```python
from build123d import *

# Parameters (mm, degrees)
F1_DEPTH  = 76.2
F2_R      = 26.962809
F3_DEPTH  = 63.798865
F5_DEPTH  = 127
F7_DEPTH  = 127
F8_R      = 8.119413
F9_DEPTH  = 48.922082
F10_R     = 9.932107
F11_DEPTH = 52.600686


with BuildPart() as f1:
    # F0 (on Front) → F1 (new body)
    with BuildSketch(Plane.XZ):
        Polygon((-32.091218, -26.459824), (-32.091218, -51.57762), (56.808782, -51.57762), (56.808782, -26.17762), (31.408782, -26.17762), (31.408782, 37.32238), (56.808782, 37.32238), (56.808782, 62.72238), (-32.389083, 62.72238), (-32.091218, 35.914471), (-7.385746, 36.188975), (-6.692785, -26.17762), align=None)
    extrude(amount=F1_DEPTH)

    # F2 (on face) → F3 (cut, through all)
    with BuildSketch(Plane.YZ.offset(31.408782)):
        with Locations((-38.1, 5.57238)):
            Circle(F2_R)
    extrude(amount=-F3_DEPTH, mode=Mode.SUBTRACT)

    # F4 (on face) → F5 (join)
    with BuildSketch(Plane.XY.offset(62.72238)):
        Polygon((5.720465, -23.600314), (7.3049, -48.921082), (38.345255, -48.921082), (38.345255, -23.600314), align=None)
    extrude(amount=F5_DEPTH)

    # F6 (on face) → F7 (join)
    with BuildSketch(Plane.XY.offset(62.72238)):
        Polygon((-2.503503, -46.93903), (-10.301619, -21.702323), (-23.880914, -20.912418), (-23.880914, -46.93903), align=None)
    extrude(amount=F7_DEPTH)

    # F8 (on face) → F9 (cut, through all)
    with BuildSketch(Plane.XZ.offset(48.921082)):
        with Locations((21.437701, 170.965254)):
            Circle(F8_R)
    extrude(amount=-F9_DEPTH, mode=Mode.SUBTRACT)

    # F10 (on face) → F11 (cut, through all)
    with BuildSketch(Plane(origin=(0, -23.600314, 0), x_dir=(-1, 0, 0), z_dir=(0, 1, 0))):
        with Locations((-22.03286, 84.947929)):
            Circle(F10_R)
    extrude(amount=-F11_DEPTH, mode=Mode.SUBTRACT)


solid = f1.part
```
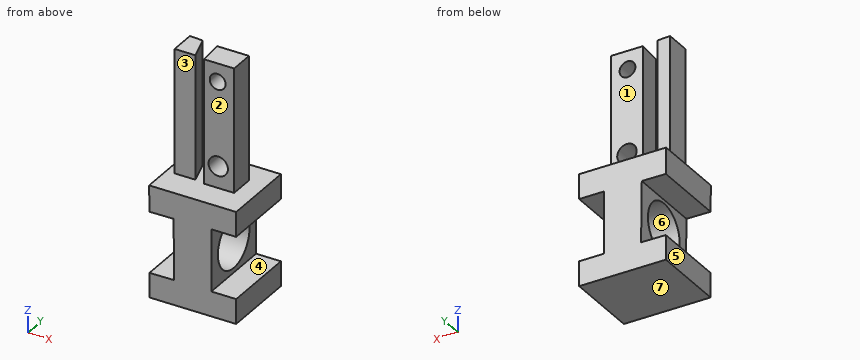
The listing builds one solid part. Answer for the finished solid, in the listing's coordinates (mm). Face numbers are marked on the shaded views. A direction names the side the tool comes from. Round coordinates to 2 decimals unless told otherwise and drop trailing zeros. Write each loop counter-clockwise with the first axis right and the second up, starting at its lowest first coordinate (ties: lowest second). Pieces come first, ordered by that corner, then holes. Notation, with made-up numbers: (12, -7.75) -> (46, -7.75) arc R15 ccw to (46, 11.25) -> close; hole circle Ø5 at (32, -16.5). An arc over 180 degrees is marked (long way). Answer as a JSON object with one key per item and string values. Group by question number.
Q1. Section A-A (z = 144.5) is taken. Write down the section's boundary in (x, y).
Q2. Section C-C (y = -18) is taken. Write down the section's boundary in (x, z).
Q3. Section B-B (y = -38.1) is taken. Write down the section's boundary in (x, z).
Q4. Section D-D (z = 89) is taken. Write down the section's boundary in (x, y).
Q5. Straight lines are drawn through the part: line 1 along Z through (x, y) = (-7.5, -43); line 2 along Z through (x, y) = (16, -44); line 3 along Z through (x, y) = (-28, -8.5). For each, find the intervals that lie inside material, in ascending order.
Q6. Which of the six approach directions +Z, -Z, +X, -X, +Y, -Y give full straight-line access (tool end or side, diameter ignored) to the marked faces 1, 2, 3 and 4?
Q7. Each of these flat-tipped pins is pushed along its axis until it touches: pin 1 Ø1 at (x, z) = (1, -21) entering from +Y; pin 2 Ø1.5 at (x, z) = (12.5, 150) entering from -Y; pin 3 Ø12.5 at (y, z) = (-40.5, 156) entering from +X; pin 4 Ø5 at (x, z) = (-6.5, 109.5) entering from -Y. Where does it stop, or does it pass through?
Q8. Determine the mould class of the marked faces 5, 6 and 7 for opening direction Z: pulls with the +Z half, pulls with the -Z half, needs draft (parallel to the pull), parting line crosses it, or undercut.
Check values:
{
 "1": {"outline": "(-23.88, -46.94) -> (-2.5, -46.94) -> (-10.3, -21.7) -> (-23.88, -20.91) -> close; (5.72, -23.6) -> (7.3, -48.92) -> (38.35, -48.92) -> (38.35, -23.6) -> close"},
 "2": {"outline": "(-32.39, 62.72) -> (-32.09, 35.91) -> (-7.39, 36.19) -> (-7.25, 23.54) -> (31.41, 23.54) -> (31.41, 37.32) -> (56.81, 37.32) -> (56.81, 62.72) -> close; (-32.09, -51.58) -> (56.81, -51.58) -> (56.81, -26.18) -> (31.41, -26.18) -> (31.41, -12.4) -> (-6.85, -12.4) -> (-6.69, -26.18) -> (-32.09, -26.46) -> close"},
 "3": {"outline": "(-32.39, 62.72) -> (-32.09, 35.91) -> (-7.39, 36.19) -> (-7.35, 32.54) -> (31.41, 32.54) -> (31.41, 37.32) -> (56.81, 37.32) -> (56.81, 62.72) -> (38.35, 62.72) -> (38.35, 189.72) -> (6.63, 189.72) -> (6.63, 62.72) -> (-5.23, 62.72) -> (-5.23, 189.72) -> (-23.88, 189.72) -> (-23.88, 62.72) -> close; (-32.09, -51.58) -> (56.81, -51.58) -> (56.81, -26.18) -> (31.41, -26.18) -> (31.41, -21.39) -> (-6.75, -21.39) -> (-6.69, -26.18) -> (-32.09, -26.46) -> close; hole circle Ø19.86 at (22.03, 84.95); hole circle Ø16.24 at (21.44, 170.97)"},
 "4": {"outline": "(-23.88, -46.94) -> (-2.5, -46.94) -> (-10.3, -21.7) -> (-23.88, -20.91) -> close; (5.72, -23.6) -> (7.3, -48.92) -> (12.96, -48.92) -> (12.96, -23.6) -> close; (31.1, -48.92) -> (38.35, -48.92) -> (38.35, -23.6) -> (31.1, -23.6) -> close"},
 "5": {"line 1": "-51.58 to -26.19, 36.19 to 189.72", "line 2": "-51.58 to -20.74, 31.88 to 77.06, 92.84 to 164.94, 176.99 to 189.72", "line 3": "-51.58 to -26.41, 35.96 to 62.72"},
 "6": {"face 1": "+Z, +X, +Y", "face 2": "+Z, +X, -X, -Y", "face 3": "+Z, -X, -Y", "face 4": "+X, +Y, -Y"},
 "7": {"pin 1": "y = 0", "pin 2": "y = -48.92", "pin 3": "x = 38.35", "pin 4": "y = -46.94"},
 "8": {"face 5": "needs draft", "face 6": "undercut", "face 7": "pulls with the -Z half"}
}
